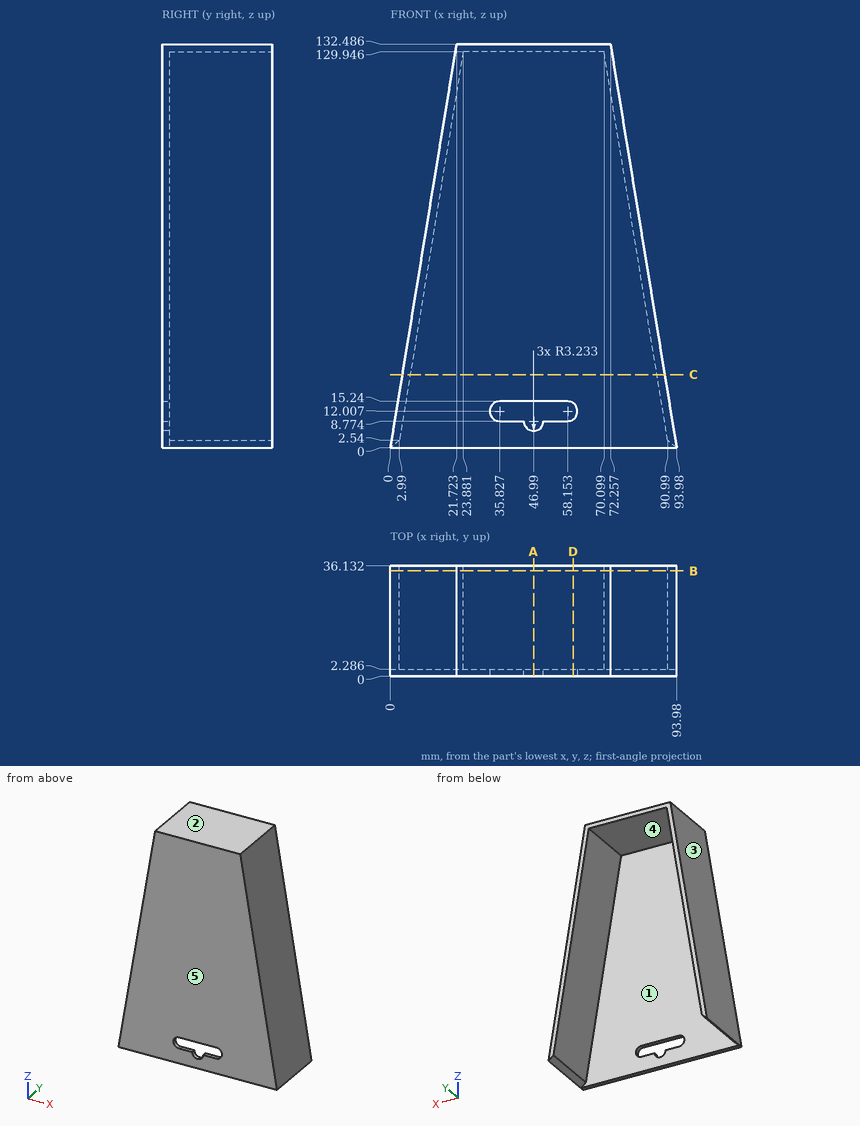
Geometry check sheet. Reference: drawing and pictorial views, mm from the part's lowest x, y, z. A direction names the side the tool comes from. Give positions to 0.01 mm unless a question says otherwise; leave off trailing zeros. Order: outer loops, then holes, each group sorted by start corner. A loop starts at its lowest first (then second) coordinate and runs counter-clockwise, first axis right, second up.
1. Section check A-A, the plane x = 46.99. Enter the section's corners in (y, z) (1 decimal).
2. Section check C-C, the plane z = 24. Enter the section's corners in (x, y) (1 decimal).
3. Section check D-D, the plane x = 60. Enter the section's corners in (y, z) (1 decimal).
4. Release check for a two-part mould opening along X. For the marked faces 3, 4 and 5 record: pulls with the +X half, pulls with the -X half, needs draft (parallel to the pull), parting line crosses it, or undercut.
5. Access from +Z, -Z, +X, -X, +Y, -Y to the whole of each face (thin tool, end or side, straight path). Record for the marked faces 1 and 2.
6. Section check B-B, the plane y = 34.5. Enter the section's corners in (x, z).
7. Thickness scan on L1, parallel to Y at x = 75, z = 11 (1 decimal); L2, parallel to Z at x = 55, y = 10.5; L3, parallel to X at y = 34.5, z = 81.5. Record the ranges inside material, lowest first.
8. Gauge pin test, flat ends, axial feed: pin 1 Ø3 at (x, y) = (45, 19) entering from -Z; pin 2 Ø12 at (x, z) = (57.5, 38) entering from +Y; pin 3 Ø1 at (y, z) = (28, 62.5) entering from +X; pin 4 Ø2.5 at (x, y) = (49.5, 1) entering from -Z. Record the tip position at first contact, or that the pin passes through.
Values follow:
1. outline: (0, 0) - (2.3, 0) - (2.3, 5.5) - (0, 5.5) - close; (0, 15.2) - (2.3, 15.2) - (2.3, 129.9) - (36.1, 129.9) - (36.1, 132.5) - (0, 132.5) - close
2. outline: (3.9, 0) - (90, 0) - (90, 36.1) - (87.5, 36.1) - (87.5, 2.3) - (6.5, 2.3) - (6.5, 36.1) - (3.9, 36.1) - close
3. outline: (0, 0) - (2.3, 0) - (2.3, 9.4) - (0, 9.4) - close; (0, 14.7) - (2.3, 14.7) - (2.3, 129.9) - (36.1, 129.9) - (36.1, 132.5) - (0, 132.5) - close
4. face 3: pulls with the -X half
4. face 4: undercut
4. face 5: needs draft
5. face 1: -Z, +Y
5. face 2: +Z, +X, -X, +Y, -Y
6. outline: (0, 0) - (2.99, 2.54) - (23.88, 129.95) - (70.1, 129.95) - (90.99, 2.54) - (93.98, 0) - (72.26, 132.49) - (21.72, 132.49) - close
7. L1: y = 0 to 2.3
7. L2: z = 129.95 to 132.49
7. L3: x = 13.36 to 15.94, 78.04 to 80.62
8. pin 1: stops at z = 129.95
8. pin 2: stops at y = 2.29
8. pin 3: stops at x = 83.81
8. pin 4: stops at z = 0
